Source: CAD feature listing. Evaluate the final solid. Frame: model axes, mm. Coordinates: 2 decimals unless noted, no trailing zeros. Loops run counter-clockwise (first coordinate to the right, second up) from the corner with the lowest first, then second, coordinate; pieces in that order, holes last. Notation, with made-up numbers: M 26.25,-29.5 L 41.25,-29.5 A19 cw 41.25,0.5 Z; hole C 59.25,59 d2. An arc over 180 degrees is marked long. One line per question, with ' | ' between items. Start each with the question number.
1. Pin query (flat end, axial travel): P1, Ø6, axis at x = 138.5, y = -116, coming from the -Z side. Return the tip coordinate at first contact, or that it passes through.
2. Section query A-A, the plane y = -8. Output: boundary loops of the cut face in (x, z).
3. Ray query, probe 1 along X at (y, z) = (89, 243.5); probe 2 along X at (y, z) = (10.5, 35); probe 3 along Y at (x, z) = (72.5, 251). Return the intervals inside material, ascending.
4. Section query B-B, the plane z = 375. Output: boundary loops of the cut face in (x, y).
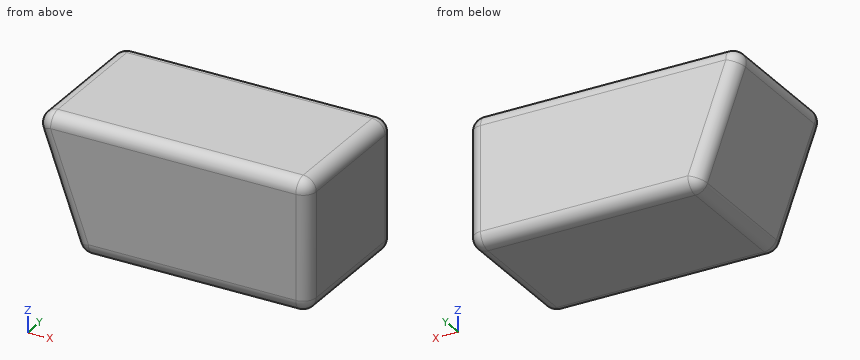
```python
from build123d import *

# Parameters (mm, degrees)
F1_DEPTH = 225
F2_R     = 40


with BuildPart() as f1:
    # F0 (on Front) → F1 (new body, symmetric)
    with BuildSketch(Plane.XZ):
        Polygon((0, 400), (145.588094, 0), (850, 0), (850, 400), align=None)
    extrude(amount=F1_DEPTH, both=True)

    # F2
    f2_edges = [f1.edges().sort_by_distance(p)[0] for p in [
        (497.794047, -225, 0),
        (145.588094, 0, 0),
        (497.794047, 225, 0),
        (850, 0, 0),
        (72.794047, -225, 200),
        (850, 225, 200),
        (850, 0, 400),
        (850, -225, 200),
        (425, 225, 400),
        (0, 0, 400),
        (425, -225, 400),
        (72.794047, 225, 200),
    ]]
    fillet(f2_edges, radius=F2_R)


solid = f1.part
```
Taken from the geometry:
1) P1: z = 16.13
2) outline: M 19.54,346.32 L 136.01,26.32 A40 ccw 173.6,0 L 810,0 A40 ccw 850,40 L 850,360 A40 ccw 810,400 L 57.13,400 A40 ccw Z
3) probe 1: 56.96 to 850 | probe 2: 132.85 to 849.69 | probe 3: -217.84 to 217.84
4) outline: M 20.04,-185 A37.08 ccw 57.13,-222.08 L 810,-222.08 A37.08 ccw 847.08,-185 L 847.08,185 A37.08 ccw 810,222.08 L 57.13,222.08 A37.08 ccw 20.04,185 Z
